Check sheet for the modelled part. Datum: model origin and axes. Units: mm. Face numbers are marked on the shaded views. A direction names the side the tool comes from. Give positions to 0.01 mm unless a question says otherwise; leave off trailing zeros. Order: outer loops, then holes, each group sorted by start corner. A loop starts at its lowest first (then second) coordinate and runs counter-clockwise, first axis right, second up. Notation, with made-up numbers: (80.5, -30) -> (139.5, -30) arc R32 cw to (139.5, 9) -> close; hole circle Ø11 at (-37, -30.5). An arc over 180 degrees is marked (long way). One line per question, with ' | ' between items.
```python
from build123d import *

# Parameters (mm, degrees)
F0_W     = 47.244
F0_H     = 25.4
F1_DEPTH = 12.7
F2_R     = 1.9558
F3_DEPTH = 12.7
F4_R     = 3.3528
F5_DEPTH = 4.064
F7_DEPTH = 25.4
F8_W     = 38.1
F8_H     = 10.16
F9_DEPTH = 12.7


with BuildPart() as f1:
    # F0 (on Front) → F1 (new body)
    with BuildSketch(Plane.XZ):
        with Locations((-20.444557, 9.059154)):
            Rectangle(F0_W, F0_H)
    extrude(amount=F1_DEPTH)

    # F2 (on face) → F3 (cut, through all)
    with BuildSketch(Plane(origin=(0, 0, 0), x_dir=(-1, 0, 0), z_dir=(0, 1, 0))):
        with Locations((5.712557, 2.709154)):
            Circle(F2_R)
        with Locations((35.176557, 2.709154)):
            Circle(F2_R)
    extrude(amount=-F3_DEPTH, mode=Mode.SUBTRACT)

    # F4 (on face) → F5 (cut)
    with BuildSketch(Plane(origin=(0, 0, 0), x_dir=(-1, 0, 0), z_dir=(0, 1, 0))):
        with Locations((5.712557, 2.709154)):
            Circle(F4_R)
        with Locations((35.176557, 2.709154)):
            Circle(F4_R)
    extrude(amount=-F5_DEPTH, mode=Mode.SUBTRACT)

    # F6 (on face) → F7 (cut)
    with BuildSketch(Plane.YZ.offset(3.177443)):
        with BuildLine():
            ThreePointArc((-6.35, 19.679154), (-8.47132, 14.557834), (-3.35, 16.679154))
            ThreePointArc((-3.35, 16.679154), (-4.22868, 18.800474), (-6.35, 19.679154))
        make_face()
    extrude(amount=-F7_DEPTH, mode=Mode.SUBTRACT)

    # F8 (on face) → F9 (cut, through all)
    with BuildSketch(Plane(origin=(0, 0, 0), x_dir=(-1, 0, 0), z_dir=(0, 1, 0))):
        with Locations((25.016557, 16.679154)):
            Rectangle(F8_W, F8_H)
    extrude(amount=-F9_DEPTH, mode=Mode.SUBTRACT)


solid = f1.part
```
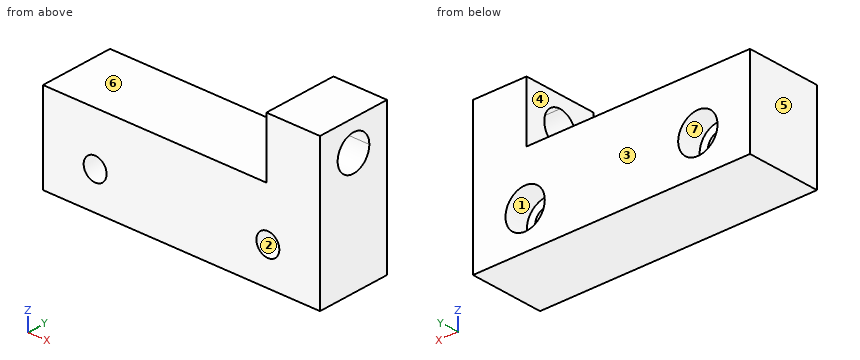
Q1. Section check D-D (y = -11.75). Enter the section's corners in (x, z).
Result sheet:
outline: (-44.07, -3.64) -> (3.18, -3.64) -> (3.18, 21.76) -> (-5.97, 21.76) -> (-5.97, 11.6) -> (-44.07, 11.6) -> close; hole circle Ø3.91 at (-35.18, 2.71); hole circle Ø3.91 at (-5.71, 2.71)
Q2. Depth check by flat-ended pin: pin 1 Ø2 at (y, z) = (-2.5, 12) entering from -X; pin 2 Ø5 at (y, z) = (-8, 15) entering from -X; pin 3 Ø3.5 at (x, z) = (-35.5, 1.5) entering from +Y. Enter the tip coordinate at first touch or a pass-through.
Result sheet:
pin 1: stops at x = -44.07 | pin 2: stops at x = -5.97 | pin 3: stops at y = -4.06
Q3. Thickness scan on line 1 (X direction, y = -9.75, z = 2.75); line 2 (Z direction, x = -1.75, y = -6.35); line 3 (X direction, y = -7, z = 3.5). Record the ranges inside material, lowest first.
Result sheet:
line 1: x = -44.07 to -37.13, -33.22 to -7.67, -3.76 to 3.18 | line 2: z = -3.64 to 13.68, 19.68 to 21.76 | line 3: x = -44.07 to -36.97, -33.39 to -7.5, -3.92 to 3.18
Q4. Access from +Z, -Z, +X, -X, +Y, -Y to the whole of each face (thin tool, end or side, straight path). Record for the marked faces 5, 6 and 7.
Result sheet:
face 5: +Z, -Z, -X, +Y, -Y | face 6: +Z, -X, +Y, -Y | face 7: +Y
Q5. Mould release check, pull along X, two halves, no side actions. Record for the marked faces 1, 2, 3 and 4: pulls with the +X half, pulls with the -X half, needs draft (parallel to the pull), parting line crosses it, or undercut.
Result sheet:
face 1: undercut | face 2: undercut | face 3: needs draft | face 4: pulls with the -X half
Q6. Section check A-A (z = 4). Enter the section's corners in (x, y), and give its area (3 significant figures).
Result sheet:
outline: (-44.07, -12.7) -> (-36.65, -12.7) -> (-36.65, -4.06) -> (-38.27, -4.06) -> (-38.27, 0) -> (-44.07, 0) -> close; (-33.71, -12.7) -> (-7.18, -12.7) -> (-7.18, -4.06) -> (-8.81, -4.06) -> (-8.81, 0) -> (-32.08, 0) -> (-32.08, -4.06) -> (-33.71, -4.06) -> close; (-4.24, -12.7) -> (3.18, -12.7) -> (3.18, 0) -> (-2.62, 0) -> (-2.62, -4.06) -> (-4.24, -4.06) -> close | area: 499 mm2
Q7. Section check B-B (y = -1). Enter the section's corners in (x, z), and give its area (3 significant figures).
Result sheet:
outline: (-44.07, -3.64) -> (3.18, -3.64) -> (3.18, 21.76) -> (-5.97, 21.76) -> (-5.97, 11.6) -> (-44.07, 11.6) -> close; hole circle Ø6.71 at (-35.18, 2.71); hole circle Ø6.71 at (-5.71, 2.71) | area: 742 mm2
Q8. Section check C-C (x = -30.5). Enter the section's corners in (y, z), and give its area (3 significant figures).
Result sheet:
outline: (-12.7, -3.64) -> (0, -3.64) -> (0, 11.6) -> (-12.7, 11.6) -> close | area: 194 mm2
